Could you check a few things on this drawing? It's one solid part, dimensions in mm from its lowest x, y, z. A direction names the side the tool comes from. Round coordinates to 2 decimals unless told otherwise and drop trailing zeros. Write each loop counter-clockwise with the first axis right and the second up, starting at its lowest first coordinate (ties: lowest second). Pieces come first, ordered by that corner, then holes. Notation, with made-up numbers: (30.5, -7.5) - (56.5, -7.5) arc R18 ccw to (56.5, 15.5) - close; hole circle Ø11 at (-8.75, 54.25). An arc over 180 degrees is marked (long way). Write item = value, one per line. Start each with the question number.
Item 1: Thinking about a two-plate mould opening in Y: for the marked faces 1, 2, 3 and 4, which applies, pulls with the +Y half, pulls with the -Y half, needs draft (parallel to the pull), parting line crosses it, or undercut?
Item 2: If we section it at C-C (z = 12.7): Give the number of separate pieces and of enclosed holes in the cut face, and give its area (3 significant figures).
Item 3: If we section it at B-B (y = 18.5): Please give me the cut outline in (x, z), and give its area (3 significant figures).
Item 4: If I drill on line 1 along Z through (x, y) = (69.85, 46.75); line 2 along X through (y, z) = (34, 5); line 3 along X through (y, z) = (22, 2.5) (1 decimal), over which ranges is the centre line in solid material (lowest first)? Write a range as [from, to].
Item 5: Which directions (+Z, -Z, +X, -X, +Y, -Y) give clear straight access to the entire face, cutting with the end or side of a thin tool? Please do the marked faces 5, 6 and 7.
Item 6: For P1, Ø1, axis at y = 19, z = 4, coming from the -X side; P2, Ø10, axis at x = 72, z = 7.5, coming from the -Y side; P3, Ø9, axis at x = 38.1, y = 17.46, coming from the -Z side; P4, Ø6, axis at y = 12.5, z = 21, coming from the +X side, each with a flat end and sliding along its axis, tell me the tip position at first contact or that it passes through.
Item 7: If we section it at A-A (x = 6.35): Please give me the cut outline in (y, z), and give its area (3 significant figures).
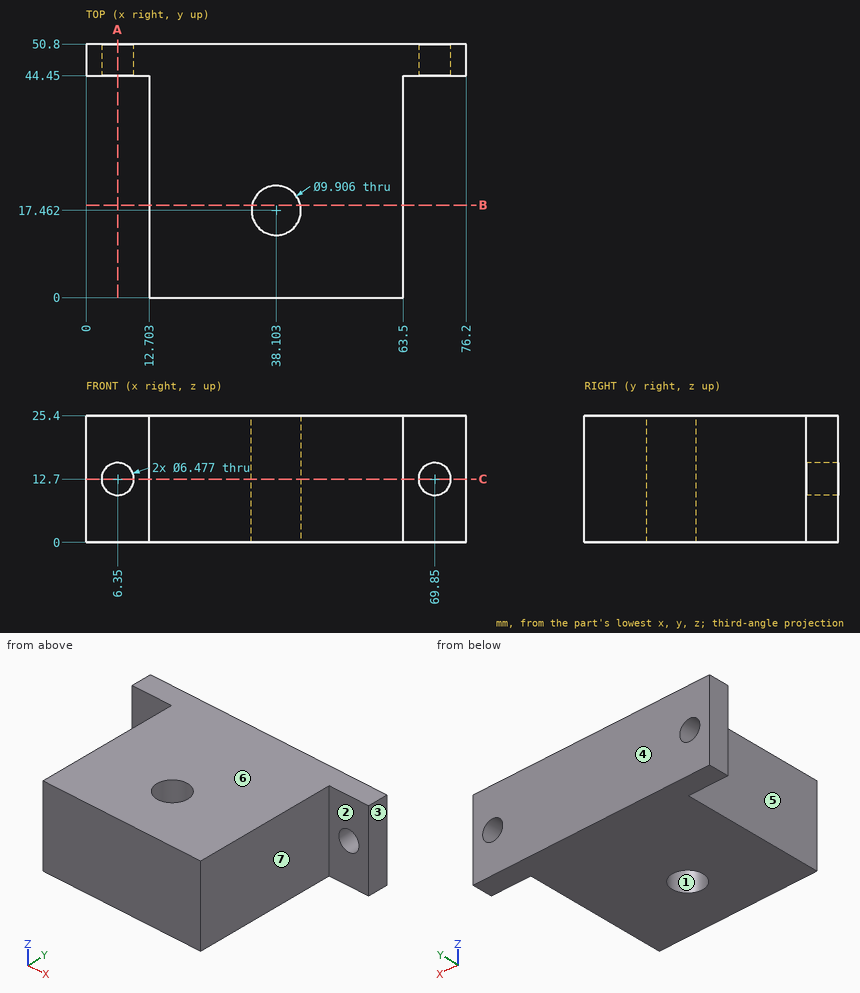
Reply:
q1.face_1 = undercut
q1.face_2 = pulls with the -Y half
q1.face_3 = needs draft
q1.face_4 = pulls with the +Y half
q2.separate_pieces = 3
q2.enclosed_holes = 1
q2.area = 2,580 mm2
q3.outline = (12.7, 0) - (33.26, 0) - (33.26, 25.4) - (12.7, 25.4) - close; (42.95, 0) - (63.5, 0) - (63.5, 25.4) - (42.95, 25.4) - close
q3.area = 1,040 mm2
q4.line_1 = [0, 9.46], [15.94, 25.4]
q4.line_2 = [12.7, 63.5]
q4.line_3 = [12.7, 36.1], [40.1, 63.5]
q5.face_5 = +Z, -Z, -X, -Y
q5.face_6 = +Z, +X, -X, +Y, -Y
q5.face_7 = +Z, -Z, +X, -Y
q6.P1 = 12.7
q6.P2 = 44.45
q6.P3 = through
q6.P4 = 63.5
q7.outline = (44.45, 0) - (50.8, 0) - (50.8, 9.46) - (44.45, 9.46) - close; (44.45, 15.94) - (50.8, 15.94) - (50.8, 25.4) - (44.45, 25.4) - close
q7.area = 120 mm2
